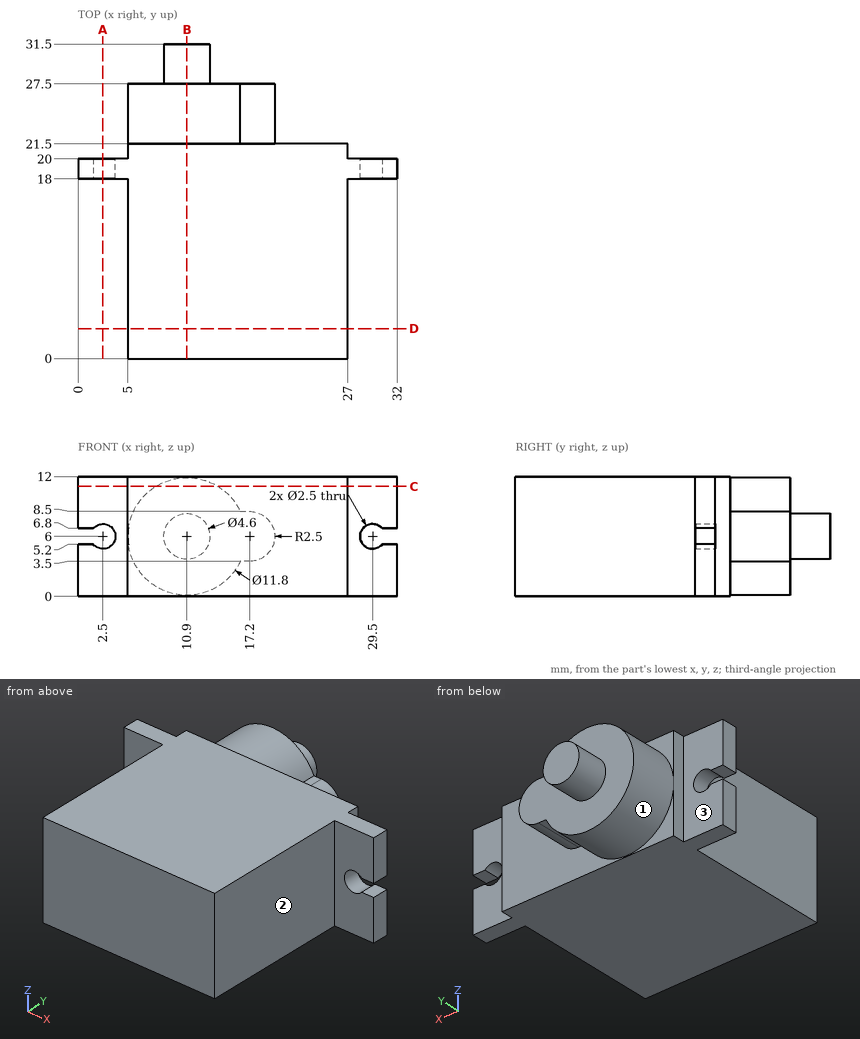
Input: dimensioned drawing with shaded views. Units: mm. Origin: part minimum x, y, z. A direction names the side the tool comes from. Give positions to 0.01 mm unless a question says otherwise; leave off trailing zeros. Order: outer loops, then holes, each group sorted by start corner. A loop starts at its lowest first (then second) coordinate and runs counter-clockwise, first axis right, second up. Notation, with made-up numbers: (36, 44.5) -> (48, 44.5) arc R7 ccw to (48, 55.5) -> close; hole circle Ø3 at (64, -19). An arc over 180 degrees is marked (long way). Answer as a JSON object with one key per item and string values.
Q1. Material intervals for probe 1 along X at (y, z) = (5.5, 8.5); probe 2 along Y at (x, z) = (7, 9.25); probe 3 along Y at (x, z) = (17, 11), sorted ascending.
Entries:
{"probe 1": "x = 5 to 27", "probe 2": "y = 0 to 27.5", "probe 3": "y = 0 to 21.5"}
Q2. Section C-C (z = 11). Output: boundary loops of the cut face in (x, y).
Entries:
{"outline": "(0, 18) -> (5, 18) -> (5, 0) -> (27, 0) -> (27, 18) -> (32, 18) -> (32, 20) -> (27, 20) -> (27, 21.5) -> (14.03, 21.5) -> (14.03, 27.5) -> (7.77, 27.5) -> (7.77, 21.5) -> (5, 21.5) -> (5, 20) -> (0, 20) -> close"}
Q3. Section B-B (x = 10.9). Output: boundary loops of the cut face in (y, z).
Entries:
{"outline": "(0, 0) -> (21.5, 0) -> (21.5, 0.1) -> (27.5, 0.1) -> (27.5, 3.7) -> (31.5, 3.7) -> (31.5, 8.3) -> (27.5, 8.3) -> (27.5, 11.9) -> (21.5, 11.9) -> (21.5, 12) -> (0, 12) -> close"}
Q4. Access query for the marked faces 1, 2 and 3. Directions: +Z, -Z, +X, -X, +Y, -Y. A direction counts if a zero-diameter tool reaches every point of the face in a straight line with its end or side. Return the directions, or none.
Entries:
{"face 1": "+Y", "face 2": "+Z, -Z, +X, -Y", "face 3": "+Z, -Z, -X, +Y"}
Q5. Section A-A (x = 2.5). Output: boundary loops of the cut face in (y, z), plus the area to 3 significant figures.
Entries:
{"outline": "(18, 0) -> (20, 0) -> (20, 4.75) -> (18, 4.75) -> close; (18, 7.25) -> (20, 7.25) -> (20, 12) -> (18, 12) -> close", "area": "19.0 mm^2"}
Q6. Section D-D (y = 3). Output: boundary loops of the cut face in (x, z).
Entries:
{"outline": "(5, 0) -> (27, 0) -> (27, 12) -> (5, 12) -> close"}
Q7. First-contact query: pin 1 (3.5 mm diameter, centred on x = 29.5, z = 6, fed in from -Y); pin 2 (5 mm diameter, centred on y = 8, z = 4, fed in from +X); pin 3 (10 mm diameter, centred on x = 16, y = 27, fed in from +Z). Flat tips, straight axial feed; report the tip coordinate or a pass-through.
Entries:
{"pin 1": "stops at y = 18", "pin 2": "stops at x = 27", "pin 3": "stops at z = 11.9"}
